Input: part model. Units: mm. Frame: model coordinates. A direction names the side the tool comes from. Round coordinates to 2 decimals unless told otherwise and drop trailing zeros. Order: outer loops, then holes, each group sorted by start corner. A loop starts at its lowest first (then second) coordinate and runs counter-clockwise, first axis right, second up. Notation, with made-up numbers: (-39, 74.25) -> (-33, 74.25) arc R17 cw to (-33, 96.25) -> close; hole circle Ø5 at (71.25, 27.5). An arc over 180 degrees is marked (long way). Use a Markdown table: item, result.
from build123d import *

# Parameters (mm, degrees)
BOSS_EXTRUDE1_DEPTH = 50.385
SKETCH3_R           = 1.95
BOSS_EXTRUDE2_DEPTH = 3.175


with BuildPart() as part:
    # Sketch1 → Boss-Extrude1 (new body)
    with BuildSketch(Plane.XY):
        Polygon((3.608439182, 0), (1.804219591, 3.125), (-1.804219591, 3.125), (-3.608439182, 0), (-1.804219591, -3.125), (1.804219591, -3.125), align=None)
    extrude(amount=BOSS_EXTRUDE1_DEPTH)

    # Sketch3 → Boss-Extrude2 (add)
    with BuildSketch(Plane.XY.offset(50.385)):
        with Locations(Location((0, 0, 0), (0, 0, 270))):
            Circle(SKETCH3_R)
    extrude(amount=BOSS_EXTRUDE2_DEPTH)


solid = part.part
1) Cut plane A-A on x = 0. Return loops of the section in (y, z) (3 decimals), and give its area (3 significant figures).
Answer key:
| item | result |
|---|---|
| outline | (-3.125, 0) -> (3.125, 0) -> (3.125, 50.385) -> (1.95, 50.385) -> (1.95, 53.56) -> (-1.95, 53.56) -> (-1.95, 50.385) -> (-3.125, 50.385) -> close |
| area | 327 mm^2 |
2) Ray query, probe 1 along Z at (x, y) = (-3, -0.75) (3 decimals); probe 2 along X at (y, z) = (1.25, 30); probe 3 along Y at (x, z) = (3.25, 33). Return the intervals inside material, ascending.
Answer key:
| item | result |
|---|---|
| probe 1 | z = 0 to 50.385 |
| probe 2 | x = -2.89 to 2.89 |
| probe 3 | y = -0.62 to 0.62 |
3) Cut plane D-D on x = -2.5. Return loops of the section in (y, z) (3 decimals), and give its area (3 significant figures).
Answer key:
| item | result |
|---|---|
| outline | (-1.92, 0) -> (1.92, 0) -> (1.92, 50.385) -> (-1.92, 50.385) -> close |
| area | 193 mm^2 |
4) Cut plane B-B on y = -0.75. Return loops of the section in (x, z) (3 decimals).
Answer key:
| item | result |
|---|---|
| outline | (-3.175, 0) -> (3.175, 0) -> (3.175, 50.385) -> (1.8, 50.385) -> (1.8, 53.56) -> (-1.8, 53.56) -> (-1.8, 50.385) -> (-3.175, 50.385) -> close |
5) Contact query for flat-ended pins moving along their axis: P1, Ø3, axis at y = 0, z = 22.5, coming from the -X side; P2, Ø2, axis at x = -2, y = -1, coming from the +Z side. Output: stop coordinate, or through.
Answer key:
| item | result |
|---|---|
| P1 | stops at x = -3.61 |
| P2 | stops at z = 53.56 |
6) Cut plane C-C on z = 38. Return loops of the section in (x, y) (3 decimals).
Answer key:
| item | result |
|---|---|
| outline | (-3.608, 0) -> (-1.804, -3.125) -> (1.804, -3.125) -> (3.608, 0) -> (1.804, 3.125) -> (-1.804, 3.125) -> close |
7) Set-up query: faces 1 (the face through (-1.187, 1.547, 51.95)), 2 (the face through (0, 0, 53.56)). Return all of +Z, -Z, +X, -X, +Y, -Y with unobstructed straight access to the full face (end or side cutting, diameter ignored); none if empty.
Answer key:
| item | result |
|---|---|
| face 1 | +Z |
| face 2 | +Z, +X, -X, +Y, -Y |
